```python
from build123d import *

# Parameters (mm, degrees)
F0_R     = 3
F1_DEPTH = 0.5
F2_R     = 2.499
F2_R_2   = 1.999
F3_DEPTH = 5.9
F4_R     = 2.75
F4_R_2   = 1.999
F5_DEPTH = 1
F7_DEPTH = 3
F8_R     = 0.14


with BuildPart() as f1:
    # F0 (on Front) → F1 (new body, symmetric)
    with BuildSketch(Plane.XZ):
        Circle(F0_R)
    extrude(amount=F1_DEPTH, both=True)

    # F2 (on face) → F3 (join)
    with BuildSketch(Plane.XZ.offset(0.5)):
        Circle(F2_R)
        Circle(F2_R_2, mode=Mode.SUBTRACT)
    extrude(amount=F3_DEPTH)

    # F4 (on face) → F5 (join)
    with BuildSketch(Plane.XZ.offset(6.4)):
        Circle(F4_R)
        Circle(F4_R_2, mode=Mode.SUBTRACT)
    extrude(amount=F5_DEPTH)

    # F6 (on face) → F7 (cut)
    with BuildSketch(Plane.XZ.offset(7.4)):
        with BuildLine():
            ThreePointArc((2.7386127875, -0.25), (2.75, 0), (2.7386127875, 0.25))
            Line((2.7386127875, 0.25), (1.983305574, 0.25))
            ThreePointArc((1.983305574, 0.25), (1.999, 0), (1.983305574, -0.25))
            Line((1.983305574, -0.25), (2.7386127875, -0.25))
        make_face()
        with BuildLine():
            Line((-2.7386127875, -0.25), (-1.983305574, -0.25))
            ThreePointArc((-1.983305574, -0.25), (-1.999, 0), (-1.983305574, 0.25))
            Line((-1.983305574, 0.25), (-2.7386127875, 0.25))
            ThreePointArc((-2.7386127875, 0.25), (-2.75, 0), (-2.7386127875, -0.25))
        make_face()
    extrude(amount=-F7_DEPTH, mode=Mode.SUBTRACT)

    # F8
    f8_edges = [f1.edges().sort_by_distance(p)[0] for p in [
        (-2.234885, -4.4, -0.25),
        (0, -6.4, 2.75),
        (0, -7.4, 2.75),
        (0, -7.4, -2.75),
        (0, -6.4, -2.75),
        (2.234885, -4.4, -0.25),
        (2.234885, -4.4, 0.25),
        (-2.234885, -4.4, 0.25),
    ]]
    fillet(f8_edges, radius=F8_R)


solid = f1.part
```
Part model, mm, in its own coordinate system. A direction names the side the tool comes from. Round coordinates to 2 decimals unless told otherwise and drop trailing zeros. Write each loop counter-clockwise with the first axis right and the second up, starting at its lowest first coordinate (ties: lowest second). Pieces come first, ordered by that corner, then holes.
Item 1: Cut at B-B, the plane x = 0. Give the cut face in (y, z), plus the area to 3 significant figures.
Results:
outline: (-7.4, -2.61) arc R0.14 ccw to (-7.26, -2.75) - (-6.54, -2.75) arc R0.14 ccw to (-6.4, -2.61) - (-6.4, -2.5) - (-0.5, -2.5) - (-0.5, -3) - (0.5, -3) - (0.5, 3) - (-0.5, 3) - (-0.5, 2.5) - (-6.4, 2.5) - (-6.4, 2.61) arc R0.14 ccw to (-6.54, 2.75) - (-7.26, 2.75) arc R0.14 ccw to (-7.4, 2.61) - (-7.4, 2) - (-0.5, 2) - (-0.5, -2) - (-7.4, -2) - close
area: 13.4 mm2
Item 2: Two-plate mould, pull along Y, no slides. Class faces 6 (the flat face through (-0.2, -7.4, 2.2)), 7 (the flat face through (0, 0.5, 0)), 8 (the cylindrical face through (2.384, -3.409, 0.751)), 9 (the cylindrical face through (-0.06, -6.89, -2.75)): +Y half, -Y half, draft (parallel to the pull), parting line (faces both ways), or undercut.
Results:
face 6: -Y half
face 7: +Y half
face 8: undercut
face 9: draft
Item 3: Probe L1, parallel to Y at x = -1.05, z = -2.3; L2, parallel to Z at x = 0, y = -2.5; L3, parallel to Y at x = -0.1, z = 1.9. List the from-to ranges inside material, lowest first.
Results:
L1: y = -7.4 to -6.4, -0.5 to 0.5
L2: z = -2.5 to -2, 2 to 2.5
L3: y = -0.5 to 0.5
Item 4: Cut at C-C, the plane z = 0. Give the cut face in (x, y).
Results:
outline: (-3, -0.5) - (-2.5, -0.5) - (-2.5, -4.4) - (-2, -4.4) - (-2, -0.5) - (2, -0.5) - (2, -4.4) - (2.5, -4.4) - (2.5, -0.5) - (3, -0.5) - (3, 0.5) - (-3, 0.5) - close
Item 5: Drop flat-ended pins along their axis: pin 1 Ø0.6 at (x, y) = (2, -5.5) entering from -Z; pin 2 Ø3 at (y, z) = (-1.5, -2) entering from +X; pin 3 Ø1.2 at (x, z) = (0, -1) entering from -Y. Give the stop position or say it passes through.
Results:
pin 1: stops at z = -1.83
pin 2: stops at x = 2.87
pin 3: stops at y = -0.5
Item 6: Which spindle directions (+Z, -Z, +X, -X, +Y, -Y) get a long thin tool onto all of the face, cutting with end or side? Do faces 1 (the cylindrical face through (-3, 0, 0)), 2 (the cylindrical face through (1.907, -3.902, 0.6)), 3 (the flat face through (0.37, -7.4, -2.12)), 4 (the cylindrical face through (0.06, -6.89, 2.75)), 5 (the flat face through (-2, -0.5, 2)). Say none if no direction does.
Results:
face 1: +Y, -Y
face 2: -Y
face 3: +Z, -Z, +X, -X, -Y
face 4: +Z, -Y
face 5: none
Item 7: Cut at D-D, the plane y = -4.25. Give the cut face in (x, z).
Results:
outline: circle Ø5 at (0, 0); hole circle Ø4 at (0, 0)
